from build123d import *

# Parameters (mm, degrees)
SKETCH1_W           = 0.2
SKETCH1_H           = 2.5
SKETCH1_W_2         = 82.6
SKETCH1_H_2         = 100
BOSS_EXTRUDE1_DEPTH = 2.23
SKETCH2_W           = 7.4
SKETCH2_H           = 3.75
SKETCH2_H_2         = 3
BOSS_EXTRUDE2_DEPTH = 4
SKETCH3_W           = 30
SKETCH3_H           = 30
CUT_EXTRUDE1_DEPTH  = 10
BOSS_EXTRUDE3_START = -82.6
SKETCH4_W           = 3
SKETCH4_H           = 2.23
BOSS_EXTRUDE3_DEPTH = 82.6
CUT_EXTRUDE2_DEPTH  = 0.5


with BuildPart() as part:
    # Sketch1 → Boss-Extrude1 (new body)
    with BuildSketch(Plane(origin=(0, 0, 0), x_dir=(1, 0, 0), z_dir=(0, 1, 0))):
        with BuildLine():
            Line((43.1, -36.85), (43.1, -37.5))
            ThreePointArc((43.1, -37.5), (44.922195524, -37.020142239), (46.5, -35.99))
            Line((46.5, -35.99), (46.5, -34.49))
            Line((46.5, -34.49), (43.1, -34.49))
            Line((43.1, -34.49), (43.1, -36.85))
        make_face()
        Polygon((41.5, -34.49), (41.3, -34.49), (41.3, -36.85), (43.1, -36.85), (43.1, -34.49), align=None)
        Polygon((45, -29.49), (41.3, -29.49), (41.3, -31.99), (41.5, -31.99), (46.5, -31.99), (46.5, -30.49), align=None)
        with Locations((41.4, -33.24)):
            Rectangle(SKETCH1_W, SKETCH1_H)
        Rectangle(SKETCH1_W_2, SKETCH1_H_2)
        Polygon((46.5, 43.01), (41.5, 43.01), (41.3, 43.01), (41.3, 40.51), (45, 40.51), (46.5, 41.51), align=None)
        with Locations((41.4, 44.26)):
            Rectangle(SKETCH1_W, SKETCH1_H)
        Polygon((41.5, 45.51), (43.1, 45.51), (43.1, 47.87), (41.3, 47.87), (41.3, 45.51), align=None)
        with BuildLine():
            ThreePointArc((43.1, 48.52), (44.922195524, 48.040142239), (46.5, 47.01))
            Line((46.5, 47.01), (46.5, 45.51))
            Line((46.5, 45.51), (43.1, 45.51))
            Line((43.1, 45.51), (43.1, 47.87))
            Line((43.1, 47.87), (43.1, 48.52))
        make_face()
        with BuildLine():
            Line((-43.1, -46.87), (-41.3, -46.87))
            Line((-41.3, -46.87), (-41.3, -44.51))
            Line((-41.3, -44.51), (-41.5, -44.51))
            Line((-41.5, -44.51), (-46.5, -44.51))
            Line((-46.5, -44.51), (-46.5, -46.01))
            ThreePointArc((-46.5, -46.01), (-44.922195524, -47.040142239), (-43.1, -47.52))
            Line((-43.1, -47.52), (-43.1, -46.87))
        make_face()
        Polygon((-41.3, -44.51), (-41.3, -39.51), (-45, -39.51), (-46.5, -40.51), (-46.5, -42.01), (-41.5, -42.01), (-41.5, -44.51), align=None)
        Polygon((-41.3, 30.49), (-41.3, 35.49), (-41.5, 35.49), (-41.5, 32.99), (-46.5, 32.99), (-46.5, 31.49), (-45, 30.49), align=None)
        with BuildLine():
            Line((-41.3, 35.49), (-41.3, 37.85))
            Line((-41.3, 37.85), (-43.1, 37.85))
            Line((-43.1, 37.85), (-43.1, 38.5))
            ThreePointArc((-43.1, 38.5), (-44.922195524, 38.020142239), (-46.5, 36.99))
            Line((-46.5, 36.99), (-46.5, 35.49))
            Line((-46.5, 35.49), (-41.5, 35.49))
            Line((-41.5, 35.49), (-41.3, 35.49))
        make_face()
    extrude(amount=BOSS_EXTRUDE1_DEPTH)

    # Sketch2 → Boss-Extrude2 (add)
    with BuildSketch(Plane(origin=(0, 2.23, 0), x_dir=(1, 0, 0), z_dir=(0, 1, 0))):
        with Locations((-25.2, -45.625)):
            Rectangle(SKETCH2_W, SKETCH2_H)
        with Locations((25.2, -45.625)):
            Rectangle(SKETCH2_W, SKETCH2_H)
        with Locations((25.2, 45.625)):
            Rectangle(SKETCH2_W, SKETCH2_H)
        with Locations((-25.2, 45.625)):
            Rectangle(SKETCH2_W, SKETCH2_H)
        with Locations((-25.2, 37.5)):
            Rectangle(SKETCH2_W, SKETCH2_H_2)
        with Locations((25.2, 37.5)):
            Rectangle(SKETCH2_W, SKETCH2_H_2)
    extrude(amount=BOSS_EXTRUDE2_DEPTH)

    # Sketch3 → Cut-Extrude1 (cut)
    with BuildSketch(Plane(origin=(0, 2.23, 0), x_dir=(1, 0, 0), z_dir=(0, 1, 0))):
        Rectangle(SKETCH3_W, SKETCH3_H)
    extrude(amount=-CUT_EXTRUDE1_DEPTH, mode=Mode.SUBTRACT)

    # Sketch4 → Boss-Extrude3 (add)
    with BuildSketch(Plane.ZY.offset(41.3).offset(BOSS_EXTRUDE3_START)):
        with BuildLine():
            ThreePointArc((-50.5, 2.23), (-51.75, 3.48), (-53, 2.23))
            Line((-53, 2.23), (-50.5, 2.23))
        make_face()
        with Locations((-51.5, 1.115)):
            Rectangle(SKETCH4_W, SKETCH4_H)
    extrude(amount=BOSS_EXTRUDE3_DEPTH)

    # Sketch5 → Cut-Extrude2 (cut)
    with BuildSketch(Plane.XZ):
        Polygon((4.640384615, -43.419230769), (4.640384615, -45.291666667), (4.070512821, -45.291666667), (4.070512821, -43.419230769), (2.198076923, -43.419230769), (2.198076923, -42.849358974), (4.070512821, -42.849358974), (4.070512821, -40.976923077), (4.640384615, -40.976923077), (4.640384615, -42.849358974), (6.512820513, -42.849358974), (6.512820513, -43.419230769), align=None)
        Polygon((1.221153846, -45.698717949), (1.221153846, -46.35), (-2.116666667, -46.35), (0.54697516, -40.651282051), (-2.03525641, -40.651282051), (-2.03525641, -40), (1.465384615, -40), (-1.198257212, -45.698717949), align=None)
        with BuildLine():
            add(Edge.make_bspline(
                [(-3.175, -44.482652244), (-3.262918211, -44.565594294), (-3.433284709, -44.726318068), (-3.671176807, -44.969181062), (-3.884395029, -45.204215059), (-4.071386431, -45.432230465), (-4.235563138, -45.650653984), (-4.373446797, -45.862117777), (-4.487450991, -46.065713922), (-4.546079998, -46.202765549), (-4.574238782, -46.268589744)],
                knots=[0, 0, 0, 0, 0.000362575, 0.000702591, 0.001019617, 0.001314251, 0.001586978, 0.001838892, 0.00207117, 0.002285828, 0.002285828, 0.002285828, 0.002285828], degree=3))
            Line((-4.574238782, -46.268589744), (-4.759955929, -46.268589744))
            add(Edge.make_bspline(
                [(-4.759955929, -46.268589744), (-4.792788221, -46.198486652), (-4.860615985, -46.053661673), (-4.986779978, -45.841364869), (-5.132525091, -45.623706079), (-5.300867212, -45.402881295), (-5.491310702, -45.177687257), (-5.702118152, -44.94759275), (-5.93585869, -44.714525691), (-6.101847246, -44.561381426), (-6.187179487, -44.482652244)],
                knots=[0, 0, 0, 0, 0.000232111, 0.000479514, 0.000739881, 0.001017698, 0.001312003, 0.001624408, 0.001953613, 0.002301902, 0.002301902, 0.002301902, 0.002301902], degree=3))
            Line((-6.187179487, -44.482652244), (-6.187179487, -44.151923077))
            add(Edge.make_bspline(
                [(-6.187179487, -44.151923077), (-6.116537815, -44.184471117), (-5.978890638, -44.247891839), (-5.781903944, -44.34935602), (-5.597143614, -44.448436612), (-5.427913951, -44.551377879), (-5.270864773, -44.651733434), (-5.129759329, -44.755968393), (-5.000056754, -44.857829341), (-4.922299946, -44.930706152), (-4.884615385, -44.966025641)],
                knots=[0, 0, 0, 0, 0.000233307, 0.000454604, 0.000664648, 0.000862076, 0.001048719, 0.001223511, 0.001388199, 0.001543075, 0.001543075, 0.001543075, 0.001543075], degree=3))
            Line((-4.884615385, -44.966025641), (-4.884615385, -38.127564103))
            Line((-4.884615385, -38.127564103), (-4.477564103, -38.127564103))
            Line((-4.477564103, -38.127564103), (-4.477564103, -44.966025641))
            add(Edge.make_bspline(
                [(-4.477564103, -44.966025641), (-4.378031962, -44.888388472), (-4.177950241, -44.732320508), (-3.858882125, -44.521130617), (-3.525108924, -44.32477265), (-3.292360048, -44.209864), (-3.175, -44.151923077)],
                knots=[0, 0, 0, 0, 0.000378565, 0.000760999, 0.001146938, 0.001539469, 0.001539469, 0.001539469, 0.001539469], degree=3))
            Line((-3.175, -44.151923077), (-3.175, -44.482652244))
        make_face()
    extrude(amount=-CUT_EXTRUDE2_DEPTH, mode=Mode.SUBTRACT)


solid = part.part
Input: part model. Units: mm. Frame: model coordinates. A direction names the side the tool comes from. Round coordinates to 2 decimals unless told otherwise and drop trailing zeros. Write each loop counter-clockwise with the first axis right and the second up, starting at its lowest first coordinate (ties: lowest second). Pieces come first, ordered by that corner, then holes.
1) Cut plane B-B (x = 36.5). Return the cut outline in (y, z), then the cut area to 3 significant figures.
2) Cut plane A-A (z = -3.5). Return the cut outline in (x, y), then the cut area to 3 significant figures.
3) Contact query for flat-ended pins moving along their axis: P1, Ø4, axis at x = 17, z = 13.5, coming from the -Y side; P2, Ø0.5, axis at y = 1, z = 47, coming from the +X side; P3, Ø1.1, axis at y = 0.5, z = 43.5, coming from the -X side; P4, Ø2, axis at x = 26.5, y = 5, coming from the -Z side. Output: stop coordinate, or through.
4) Draft query along Z for faces 6 (the flat face through (-25, 6.23, 46)), 7 (the flat face through (44, 1, 34.49)), 8 (the flat face through (1, 1, -53)). Return one class per face: pulls with the +Z half, pulls with the -Z half, needs draft (parallel to the pull), parting line crosses it, or undercut.
5) Ray query, L1, parallel to Z at x = -5.5, y = 1.5; L2, parallel to X at y = 2.5, z = -44; L3, parallel to Y at x = -18, z = -14. Return the intervals inside material, ascending.
6) Cut plane D-D (z = 22). Return the cut outline in (x, y).
7) Reachability of faces 1 (the flat face through (21.5, 4, 46)), 2 (the flat face through (44, 1, 31.99)), 3 (the flat face through (0, 1, 15)), 4 (the flat face through (0.15, 0.25, -42.81)), 5 (the flat face through (-41.3, 1, 48)) from +Z, -Z, +X, -X, +Y, -Y: full face, straight path, thin tool, end or side. Return the list, or none.
8) Cut plane C-C (z = -51.75). Return the cut outline in (x, y), then the cut area to 3 significant figures.
Geometry says:
1. outline: (0, -53) - (2.23, -53) arc R1.25 ccw to (2.23, -50.5) - (2.23, 50) - (0, 50) - close
1. area: 232 mm2
2. outline: (-41.3, 0) - (-15, 0) - (-15, 2.23) - (-41.3, 2.23) - close; (15, 0) - (41.3, 0) - (41.3, 2.23) - (15, 2.23) - close
2. area: 117 mm2
3. P1: stops at y = 0
3. P2: stops at x = 41.3
3. P3: stops at x = -41.5
3. P4: stops at z = -47.5
4. face 6: needs draft
4. face 7: undercut
4. face 8: pulls with the -Z half
5. L1: z = -53 to -15, 15 to 50
5. L2: x = -28.9 to -21.5, 21.5 to 28.9
5. L3: y = 0 to 2.23
6. outline: (-41.3, 0) - (41.3, 0) - (41.3, 2.23) - (-41.3, 2.23) - close
7. face 1: +Z, +Y
7. face 2: +X, +Y, -Y
7. face 3: +Y, -Y
7. face 4: -Y
7. face 5: +Z, +Y, -Y
8. outline: (-41.3, 0) - (41.3, 0) - (41.3, 3.48) - (-41.3, 3.48) - close
8. area: 287 mm2
